from build123d import *

# Parameters (mm, degrees)
SKETCH2_R           = 1.29
CUT_EXTRUDE1_DEPTH  = 7
BOSS_EXTRUDE1_DEPTH = 3.81


with BuildPart() as part:
    # Sketch1 → Revolve1 (revolve)
    with BuildSketch(Plane(origin=(0, 0, 0), x_dir=(0, 0, -1), z_dir=(1, 0, 0))):
        Polygon((0, 0), (0, 5.5499), (4.0513, 5.5499), (4.0513, 15.94), (8.0513, 17.575), (27.9313, 17.575), (27.9313, 6.019833944), (28.9313, 6.019833944), (28.9313, 17.575), (35.9313, 16.205000102), (35.9313, 4.73075), (36.5155, 4.73075), (36.5155, 2.4511), (37.4807, 2.4511), (37.4807, 0), align=None)
    revolve(axis=Axis((0, 0, 1000), (0, 0, -1)))

    # Sketch2 → Cut-Extrude1 (cut)
    with BuildSketch(Plane(origin=(0, 0, -35.9313), x_dir=(-1, 0, 0), z_dir=(0, 0, -1))):
        with Locations((-12.57, 0)):
            Circle(SKETCH2_R)
        with Locations((0, 9.545)):
            Circle(SKETCH2_R)
        with Locations((12.57, 0)):
            Circle(SKETCH2_R)
        with Locations((0, -9.545)):
            Circle(SKETCH2_R)
    extrude(amount=-CUT_EXTRUDE1_DEPTH, mode=Mode.SUBTRACT)

    # Sketch3 → Boss-Extrude1 (add, symmetric)
    with BuildSketch(Plane(origin=(-12.427401679, 12.427401679, 0), x_dir=(0, 0, -1), z_dir=(-0.707106781, 0.707106781, 0))):
        with BuildLine():
            Line((34.0517, 2.5019), (34.0517, -2.5019))
            ThreePointArc((34.0517, -2.5019), (32.0578, -4.4958), (30.0639, -2.5019))
            Line((30.0639, -2.5019), (30.0639, 2.5019))
            ThreePointArc((30.0639, 2.5019), (32.0578, 4.4958), (34.0517, 2.5019))
        make_face()
    extrude(amount=BOSS_EXTRUDE1_DEPTH, both=True)


solid = part.part
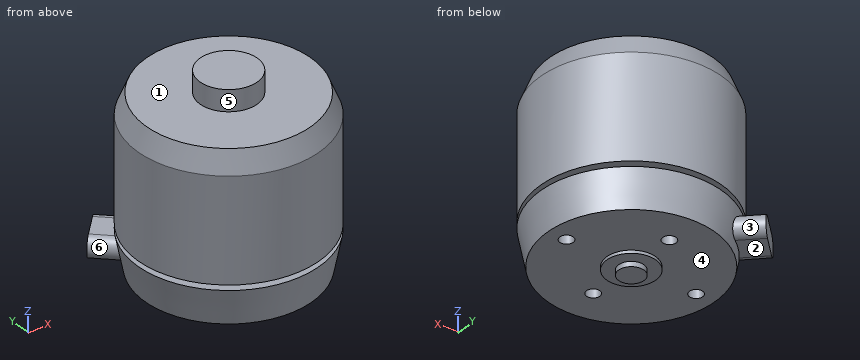
The listing builds one solid part. Answer for the finished solid, in the listing's coordinates (mm). Face numbers are marked on the shaded views. A direction names the side the tool comes from. Coordinates: 2 decimals unless noted, no trailing zeros. Write each loop counter-clockwise with the first axis right and the second up, starting at its lowest first coordinate (ties: lowest second). Pieces come first, ordered by that corner, then holes. Notation, with made-up numbers: M 22,-18.75 L 26,-18.75 A15 cw 26,0.25 Z; hole C 43.25,52 d5. An arc over 180 degrees is marked long. Put each result on its own line as item: value. Start each with the question number.
1. A cutting plane is placed at A-A on x = 0. Count the separate pieces of the cut face and the enclosed holes in it, then the cut area to 3 significant figures.
2. A cutting plane is placed at D-D on z = -3.5. Write down the section's boundary in (x, y), then the cut area to 3 significant figures.
3. For a pull along Y with two mould halves and no side action, classify the marked faces 4, 5 and 6 as pulls with the +Y half, pulls with the -Y half, needs draft (parallel to the pull), parting line crosses it, or undercut.
4. Which of the six approach directions +Z, -Z, +X, -X, +Y, -Y give full straight-line access (tool end or side, diameter ignored) to the marked faces 1, 2 and 3?
5. Consider line 1 (Z direction, x = -1, y = -13.5); line 2 (Y direction, x = 0, z = -32) (3 decimals); line 3 (Y direction, x = -12.57, z = -33.75). Determine where each line is inside the solid, lowest interval first. Write a range as from..to.
6. Flat-ended cylindrical pins translate along their axes: P1, Ø2, axis at x = -14, y = 14, coming from the +Z side; P2, Ø4, axis at x = 13, z = -28.5, coming from the +Y side; P3, Ø4, axis at x = 7, y = -12, coming from the -Z side. Find the tip coordinate at first contact, or state that the pin passes through.
7. A cutting plane is placed at C-C on z = -21. Write down the section's boundary in (x, y) (3 decimals).
Resolved:
1. separate pieces: 3
1. enclosed holes: 0
1. area: 1,100 mm2
2. outline: C 0,0 d11.1
2. area: 96.8 mm2
3. face 4: needs draft
3. face 5: parting line crosses it
3. face 6: undercut
4. face 1: +Z
4. face 2: -Z, -X, +Y
4. face 3: +Y
5. line 1: z = -35.93..-28.93, -27.93..-4.05
5. line 2: y = -16.974..-10.835, -8.255..8.255, 10.835..16.974
5. line 3: y = -10.89..-1.29, 1.29..17.6
6. P1: stops at z = -30.06
6. P2: stops at y = 13.67
6. P3: stops at z = -35.93
7. outline: C 0,0 d35.15
